from build123d import *
from build123d.topology import SkipClean

# Parameters (mm, degrees)
SKETCH1_R           = 22.1615
BOSS_EXTRUDE1_DEPTH = 12.7
SKETCH2_R           = 28.575
BOSS_EXTRUDE2_DEPTH = 3.175
BOSS_EXTRUDE3_START = 12.7
SKETCH3_R           = 22.1615
BOSS_EXTRUDE3_DEPTH = 12.7
SKETCH5_R           = 9.525
BOSS_EXTRUDE4_DEPTH = 1.5875
SKETCH6_R           = 3.175
CUT_EXTRUDE1_DEPTH  = 17.78
SKETCH8_R           = 2.413
CUT_EXTRUDE2_DEPTH  = 21.336
CUT_EXTRUDE3_START  = -22.86
SKETCH9_R           = 2.413
CUT_EXTRUDE3_DEPTH  = 22.86
BOSS_EXTRUDE6_START = 6.35
SKETCH10_R          = 2.413
BOSS_EXTRUDE6_DEPTH = 6.35
SKETCH11_R          = 2.413
BOSS_EXTRUDE7_DEPTH = 6.35


with BuildPart() as part:
    # Sketch1 → Boss-Extrude1 (new body)
    with BuildSketch(Plane.XY):
        Circle(SKETCH1_R)
        Polygon((7.478995387, 0), (3.739497694, 6.477), (-3.739497694, 6.477), (-7.478995387, 0), (-3.739497694, -6.477), (3.739497694, -6.477), align=None, mode=Mode.SUBTRACT)
    extrude(amount=BOSS_EXTRUDE1_DEPTH)

    # Sketch2 → Boss-Extrude2 (add)
    with BuildSketch(Plane.XY.offset(12.7)):
        Circle(SKETCH2_R)
        Polygon((7.478995387, 0), (3.739497694, 6.477), (-3.739497694, 6.477), (-7.478995387, 0), (-3.739497694, -6.477), (3.739497694, -6.477), align=None, mode=Mode.SUBTRACT)
    extrude(amount=BOSS_EXTRUDE2_DEPTH)

    # Sketch3 → Boss-Extrude3 (add)
    with BuildSketch(Plane(origin=(0, 0, 0), x_dir=(-1, 0, 0), z_dir=(0, 0, -1)).offset(BOSS_EXTRUDE3_START)):
        Circle(SKETCH3_R)
    extrude(amount=-BOSS_EXTRUDE3_DEPTH)

    # Sketch5 → Boss-Extrude4 (add)
    with BuildSketch(Plane.XY.offset(15.875)):
        Circle(SKETCH5_R)
        Polygon((7.478995387, 0), (3.739497694, 6.477), (-3.739497694, 6.477), (-7.478995387, 0), (-3.739497694, -6.477), (3.739497694, -6.477), align=None, mode=Mode.SUBTRACT)
    extrude(amount=BOSS_EXTRUDE4_DEPTH)

    # Sketch6 → Cut-Extrude1 (cut)
    with BuildSketch(Plane.XY):
        Circle(SKETCH6_R)
    extrude(amount=-CUT_EXTRUDE1_DEPTH, mode=Mode.SUBTRACT)

    # Sketch8 → Cut-Extrude2 (cut)
    with BuildSketch(Plane(origin=(5.60924654, -3.2385, 0), x_dir=(0, 0, 1), z_dir=(-0.8660254037844389, 0.4999999999999997, 0))):
        with Locations(Location((0, 0, 0), (0, 0, 270))):
            Circle(SKETCH8_R)
    extrude(amount=-CUT_EXTRUDE2_DEPTH, mode=Mode.SUBTRACT)

    # Sketch9 → Cut-Extrude3 (cut)
    with SkipClean():  # the faces are left unmerged after this step: merging them gives an invalid solid
        with BuildSketch(Plane(origin=(-5.60924654, 3.2385, 0), x_dir=(0, 0, -1), z_dir=(0.8660254037844386, -0.5000000000000001, 0)).offset(CUT_EXTRUDE3_START)):
            with Locations(Location((0, 0, 0), (0, 0, 270))):
                Circle(SKETCH9_R)
        extrude(amount=CUT_EXTRUDE3_DEPTH, mode=Mode.SUBTRACT)

    # Sketch10 → Boss-Extrude6 (add)
    with SkipClean():  # the faces are left unmerged after this step: merging them gives an invalid solid
        with BuildSketch(Plane(origin=(-5.60924654, 3.2385, 0), x_dir=(0, 0, 1), z_dir=(-0.8660254037844386, 0.5000000000000001, 0)).offset(BOSS_EXTRUDE6_START)):
            with Locations(Location((0, 0, 0), (0, 0, 270))):
                Circle(SKETCH10_R)
        extrude(amount=-BOSS_EXTRUDE6_DEPTH)

    # Sketch11 → Boss-Extrude7 (add)
    with SkipClean():  # the faces are left unmerged after this step: merging them gives an invalid solid
        with BuildSketch(Plane(origin=(5.60924654, -3.2385, 0), x_dir=(0, 0, -1), z_dir=(0.8660254037844388, -0.49999999999999983, 0))):
            with Locations(Location((0, 0, 0), (0, 0, 270))):
                Circle(SKETCH11_R)
        extrude(amount=BOSS_EXTRUDE7_DEPTH)


solid = part.part
Source: CAD feature listing. Evaluate the final solid. Frame: model axes, mm. A direction names the side the tool comes from. Round coordinates to 2 decimals unless told otherwise and drop trailing zeros. Order: outer loops, then holes, each group sorted by start corner. A loop starts at its lowest first (then second) coordinate and runs counter-clockwise, first axis right, second up. Notation, with made-up numbers: (40, 76.5) - (83, 76.5) arc R27 ccw to (83, 103.5) - close; hole circle Ø6 at (15.25, 50). An arc over 180 degrees is marked (long way). Use a Markdown table: item, result. Add a question column.
1. Section query A-A (z = 4.5). Return the cut outline in (x, y).
2. Section query B-B (x = 0). Return the cut outline in (y, z) (1 decimal).
3. First-contact query: pin 1 (8 mm diameter, centred on x = 18.5, z = -8, fed in from -Y); pin 2 (4 mm diameter, centred on x = 5, z = -5, fed in from -Y); pin 3 (3 mm diameter, centred on y = 3.5, z = 13, fed in from -X). Flat tips, straight axial feed; report the tip coordinate or a pass-through.
4. Mould query, pull axis X, two halves, no side actions, for faces 1 (the flat face through (0, -5, -12.7)), 2 (the cylindrical face through (-7.559, -5.796, 16.658)), 3 (the cylindrical face through (-16.323, 6.85, 0.924)), 4 (the flat face through (0, 6.477, 9)). Classes: +X half, -X half, draft (parallel to the pull), parting line (faces both ways), or undercut.
5. Line query: probe 1 along Y at (x, z) = (0, -4) (1 decimal); probe 2 along Z at (x, y) = (11.5, 20) (3 decimals); probe 3 along Z at (x, y) = (8, -18) (3 decimals). Output: solid intervals per line, ascending.
6. Set-up query: faces 5 (the flat face through (-2, -3, 0)), 6 (the flat face through (11.13, -6.38, -0.03)), 7 (the flat face through (15, -17, 12.7)). Return all of +Z, -Z, +X, -X, +Y, -Y with unobstructed straight access to the full face (end or side cutting, diameter ignored); none if empty.
Derived:
| question | item | result |
|---|---|---|
| 1 | outline | circle Ø44.32 at (0, 0); hole (-7.48, 0) - (-3.74, -6.48) - (3.74, -6.48) - (7.48, 0) - (3.74, 6.48) - (-3.74, 6.48) - close |
| 2 | outline | (-28.6, 12.7) - (-22.2, 12.7) - (-22.2, -12.7) - (-3.2, -12.7) - (-3.2, 0) - (-6.5, 0) - (-6.5, 17.5) - (-9.5, 17.5) - (-9.5, 15.9) - (-28.6, 15.9) - close; (3.2, -12.7) - (22.2, -12.7) - (22.2, 12.7) - (28.6, 12.7) - (28.6, 15.9) - (9.5, 15.9) - (9.5, 17.5) - (6.5, 17.5) - (6.5, 0) - (3.2, 0) - close |
| 3 | pin 1 | y = -16.76 |
| 3 | pin 2 | y = -21.96 |
| 3 | pin 3 | x = -28.5 |
| 4 | face 1 | draft |
| 4 | face 2 | parting line |
| 4 | face 3 | undercut |
| 4 | face 4 | undercut |
| 5 | probe 1 | -22.2 to -3.2, 3.2 to 22.2 |
| 5 | probe 2 | 12.7 to 15.875 |
| 5 | probe 3 | -12.7 to 15.875 |
| 6 | face 5 | +Z |
| 6 | face 6 | none |
| 6 | face 7 | -Z |
